The listing builds one solid part. Answer for the finished solid, in the listing's coordinates (mm). A direction names the side the tool comes from. Give positions to 0.01 mm unless a question says otherwise; leave off trailing zeros. Loops run counter-clockwise (first coordinate to the right, second up) from the corner with the lowest first, then second, coordinate; pieces in that order, holes last. Notation, with made-up numbers: M 83.5,-2.75 L 140.5,-2.75 A21 cw 140.5,33.25 Z; hole C 34.25,53.5 d7. An arc over 180 degrees is marked long. One line per item, written item: value. Start each with the question number.
Q1. Consider L1, parallel to X at y = 243, z = 31; L2, parallel to X at y = -190.5, z = 72.5; L3, parallel to Z at x = -800.1, y = 295.5 (3 decimals). Determine where each line is inside the solid, lowest interval first.
Q2. The mould has two halves that part along Y. Classify faces 5 (the flat face through (444, 4, 25.4)), 6 (the flat face through (-12, 323.85, 44)), 7 (the flat face through (-4, 313, 88.9)): +Y half, -Y half, draft (parallel to the pull), parting line (faces both ways), or undercut.
Q3. For faces 1 (the flat face through (-4, -1, 63.5)), 2 (the flat face through (857.25, -5, 44)), 3 (the flat face through (0, 4, 25.4)), 4 (the flat face through (-463.55, -4, 45)), determine the directions among +Z, -Z, +X, -X, +Y, -Y from which every point of the face is accessible in a straight line to the end or side of a thin tool.
Q4. A cutting plane is placed at B-B, the plane y = -55. Determine the outline of the cut face in (x, z), and give its area (3 significant figures).
Q5. A cutting plane is placed at A-A, the plane x = -683. Determine the outline of the cut face in (y, z), and give its area (3 significant figures).
Q6. A flat-ended cylindrical pin translates along its axis: pin 1 (4 mm diameter, centred on y = 266.7, z = 12.7, fed in from +X). Find the tip coordinate at first contact, or state that the pin passes through.
from build123d import *

# Parameters (mm, degrees)
F0_W      = 1714.5
F0_H      = 647.7
F0_W_2    = 1676.4
F0_H_2    = 609.6
F1_DEPTH  = 88.9
F2_W      = 1676.4
F2_H      = 609.6
F2_W_2    = 1638.3
F2_H_2    = 571.5
F3_DEPTH  = 63.5
F4_W      = 38.1
F4_H      = 571.5
F5_DEPTH  = 38.1
F6_R      = 3.175
F7_DEPTH  = 647.701
F8_R      = 3.175
F9_DEPTH  = 50.8
F10_R     = 3.175
F11_DEPTH = 50.8
F12_SIZE  = 6.35


with BuildPart() as f1:
    # F0 (on Top) → F1 (new body)
    with BuildSketch(Plane.XY):
        Rectangle(F0_W, F0_H)
        Rectangle(F0_W_2, F0_H_2, mode=Mode.SUBTRACT)
    extrude(amount=F1_DEPTH)

    # F2 (on face) → F3 (join)
    with BuildSketch(Plane(origin=(0, 0, 0), x_dir=(1, 0, 0), z_dir=(0, 0, -1))):
        Rectangle(F2_W, F2_H)
        Rectangle(F2_W_2, F2_H_2, mode=Mode.SUBTRACT)
    extrude(amount=-F3_DEPTH)

    # F4 (on face) → F5 (join)
    with BuildSketch(Plane.XY.offset(63.5)):
        Rectangle(F4_W, F4_H)
        with Locations((444.5, 0)):
            Rectangle(F4_W, F4_H)
        with Locations((-444.5, 0)):
            Rectangle(F4_W, F4_H)
    extrude(amount=-F5_DEPTH)

    # F6 (on face) → F7 (cut, through all)
    with BuildSketch(Plane.XZ.offset(323.85)):
        with Locations((-800.1, 38.1)):
            Circle(F6_R)
        with Locations((800.1, 38.1)):
            Circle(F6_R)
    extrude(amount=-F7_DEPTH, mode=Mode.SUBTRACT)

    # F8 (on face) → F9 (cut)
    with BuildSketch(Plane.YZ.offset(857.25)):
        with Locations((-266.7, 12.7)):
            Circle(F8_R)
        with Locations((266.7, 12.7)):
            Circle(F8_R)
    extrude(amount=-F9_DEPTH, mode=Mode.SUBTRACT)

    # F10 (on face) → F11 (cut)
    with BuildSketch(Plane(origin=(-857.25, 0, 0), x_dir=(0, -1, 0), z_dir=(-1, 0, 0))):
        with Locations((-266.7, 12.7)):
            Circle(F10_R)
        with Locations((266.7, 12.7)):
            Circle(F10_R)
    extrude(amount=-F11_DEPTH, mode=Mode.SUBTRACT)

    # F12
    f12_edges = [f1.edges().sort_by_distance(p)[0] for p in [
        (0, 304.8, 88.9),
        (838.2, 0, 88.9),
        (-838.2, 0, 88.9),
        (0, -304.8, 88.9),
    ]]
    chamfer(f12_edges, length=F12_SIZE)


solid = f1.part
Answer block:
1. L1: -857.25 to -819.15, -463.55 to -425.45, -19.05 to 19.05, 425.45 to 463.55, 819.15 to 857.25
1. L2: -857.25 to -838.2, 838.2 to 857.25
1. L3: 0 to 34.925, 41.275 to 63.5
2. face 5: undercut
2. face 6: +Y half
2. face 7: draft
3. face 1: +Z
3. face 2: +Z, -Z, +X, +Y, -Y
3. face 3: -Z
3. face 4: +Z, -Z
4. outline: M -857.25,0 L -819.15,0 L -819.15,63.5 L -838.2,63.5 L -838.2,82.55 L -844.55,88.9 L -857.25,88.9 Z; M -463.55,25.4 L -425.45,25.4 L -425.45,63.5 L -463.55,63.5 Z; M -19.05,25.4 L 19.05,25.4 L 19.05,63.5 L -19.05,63.5 Z; M 425.45,25.4 L 463.55,25.4 L 463.55,63.5 L 425.45,63.5 Z; M 819.15,0 L 857.25,0 L 857.25,88.9 L 844.55,88.9 L 838.2,82.55 L 838.2,63.5 L 819.15,63.5 Z
4. area: 10,100 mm^2
5. outline: M -323.85,0 L -285.75,0 L -285.75,63.5 L -304.8,63.5 L -304.8,82.55 L -311.15,88.9 L -323.85,88.9 Z; M 285.75,0 L 323.85,0 L 323.85,88.9 L 311.15,88.9 L 304.8,82.55 L 304.8,63.5 L 285.75,63.5 Z
5. area: 5,770 mm^2
6. pin 1: through
